```python
from build123d import *

# Parameters (mm, degrees)
SKETCH3_W           = 63
SKETCH3_H           = 49.6
BOSS_EXTRUDE1_DEPTH = 1.5
SKETCH10_W          = 2
SKETCH10_H          = 5
SKETCH10_W_2        = 1.5
BOSS_EXTRUDE2_DEPTH = 63
SKETCH11_W          = 5.5
SKETCH11_H          = 5.002720327
BOSS_EXTRUDE3_DEPTH = 4
SKETCH12_W          = 5.5
SKETCH12_H          = 5
BOSS_EXTRUDE4_DEPTH = 4


with BuildPart() as part:
    # Sketch3 → Boss-Extrude1 (new body)
    with BuildSketch(Plane.XY):
        Rectangle(SKETCH3_W, SKETCH3_H)
    extrude(amount=BOSS_EXTRUDE1_DEPTH)

    # Sketch10 → Boss-Extrude2 (add)
    with BuildSketch(Plane(origin=(31.5, 0, 0), x_dir=(0, 0, -1), z_dir=(1, 0, 0))):
        with Locations((-2.5, 27.3)):
            Rectangle(SKETCH10_W, SKETCH10_H)
        with Locations((-0.75, 27.3)):
            Rectangle(SKETCH10_W_2, SKETCH10_H)
        with Locations((1, 27.3)):
            Rectangle(SKETCH10_W, SKETCH10_H)
    extrude(amount=-BOSS_EXTRUDE2_DEPTH)

    # Sketch11 → Boss-Extrude3 (add)
    with BuildSketch(Plane(origin=(31.5, 0, 0), x_dir=(0, 0, -1), z_dir=(1, 0, 0))):
        with Locations((-0.75, 27.298639837)):
            Rectangle(SKETCH11_W, SKETCH11_H)
    extrude(amount=BOSS_EXTRUDE3_DEPTH)

    # Sketch12 → Boss-Extrude4 (add)
    with BuildSketch(Plane.ZY.offset(31.5)):
        with Locations((0.75, 27.3)):
            Rectangle(SKETCH12_W, SKETCH12_H)
    extrude(amount=BOSS_EXTRUDE4_DEPTH)


solid = part.part
```
Can you work these out from the model? Positions are in its coordinate system, mm. A direction names the side the tool comes from. Round coordinates to 2 decimals unless told otherwise and drop trailing zeros. Loops run counter-clockwise (first coordinate to the right, second up) from the corner with the lowest first, then second, coordinate; pieces in that order, holes last. Notation, with made-up numbers: M 45.5,-14 L 57.5,-14 A30 ccw 57.5,15 Z; hole C 27.5,5 d1. An arc over 180 degrees is marked long. Answer in a Markdown table with one row per item.
1. If we section it at B-B, the plane x = 7: Please give me the cut outline in (y, z).
Established:
| item | result |
|---|---|
| outline | M -24.8,0 L 24.8,0 L 24.8,-2 L 29.8,-2 L 29.8,3.5 L 24.8,3.5 L 24.8,1.5 L -24.8,1.5 Z |
2. I'm going to push flat-ended pins straight in: pin 1 Ø2 at (x, z) = (34, 1.5) entering from -Y; pin 2 Ø1.2 at (y, z) = (12.5, 0.5) entering from +X; pin 3 Ø15 at (x, y) = (-6, 2) entering from +Z; pin 4 Ø3 at (x, z) = (-13, -0.5) entering from -Y. Where does each tip first touch, or does it pass through?
Established:
| item | result |
|---|---|
| pin 1 | y = 24.8 |
| pin 2 | x = 31.5 |
| pin 3 | z = 1.5 |
| pin 4 | y = -24.8 |
3. On a 3-axis mill with a long thin cutter (end or side, diameter ignored), from which of +Z, -Z, +X, -X, +Y, -Y can I reach the whole of each face in a straight line? I mean faces 1 (the face through (0, 0, 1.5)), 2 (the face through (33, 24.797, 1)), 3 (the face through (-31.5, 0, 1)). Say none if no direction works.
Established:
| item | result |
|---|---|
| face 1 | +Z, +X, -X, -Y |
| face 2 | +Z, -Z, +X, -Y |
| face 3 | +Z, -Z, -X, -Y |
4. If we section it at C-C, the plane y = 6: Please give me the cut outline in (x, z).
Established:
| item | result |
|---|---|
| outline | M -31.5,0 L 31.5,0 L 31.5,1.5 L -31.5,1.5 Z |
5. If we section it at A-A, the plane z = 0.75: Please give me the cut outline in (x, y), plus the area to 3 significant figures.
Established:
| item | result |
|---|---|
| outline | M -35.5,24.8 L -31.5,24.8 L -31.5,-24.8 L 31.5,-24.8 L 31.5,24.8 L 35.5,24.8 L 35.5,29.8 L -35.5,29.8 Z |
| area | 3,480 mm² |
6. Please list where these lines run through material, in increasing order: line 1 (X direction, y = 0, z = 0.9); line 2 (Y direction, x = -7.5, z = -1.1); line 3 (Z direction, x = 18, y = -1). Write a range as from..to.
Established:
| item | result |
|---|---|
| line 1 | -31.5..31.5 |
| line 2 | 24.8..29.8 |
| line 3 | 0..1.5 |
